from build123d import *

# Parameters (mm, degrees)
SKETCH1_W           = 110
SKETCH1_H           = 130
BOSS_EXTRUDE1_DEPTH = 4
SKETCH2_R           = 4.5
CUT_EXTRUDE1_DEPTH  = 4
SKETCH4_R           = 2.15
CUT_EXTRUDE2_DEPTH  = 86.240835285
SKETCH5_R           = 2.15
CUT_EXTRUDE3_DEPTH  = 86.240835285


with BuildPart() as part:
    # Sketch1 → Boss-Extrude1 (new body)
    with BuildSketch(Plane.XY):
        Rectangle(SKETCH1_W, SKETCH1_H)
    extrude(amount=BOSS_EXTRUDE1_DEPTH)

    # Sketch2 → Cut-Extrude1 (cut)
    with BuildSketch(Plane.XY.offset(4)):
        with Locations((0, 34.993291231)):
            Circle(SKETCH2_R)
    extrude(amount=-CUT_EXTRUDE1_DEPTH, mode=Mode.SUBTRACT)

    # Sketch4 → Cut-Extrude2 (cut, through all)
    with BuildSketch(Plane.XY.offset(4)):
        with Locations((-45.36112854, -47.475954891)):
            Circle(SKETCH4_R)
    extrude(amount=-CUT_EXTRUDE2_DEPTH, mode=Mode.SUBTRACT)

    # Sketch5 → Cut-Extrude3 (cut, through all)
    with BuildSketch(Plane.XY.offset(4)):
        with Locations((45.36112854, -47.475954891)):
            Circle(SKETCH5_R)
    extrude(amount=-CUT_EXTRUDE3_DEPTH, mode=Mode.SUBTRACT)


solid = part.part
Geometry: final body of the model. Coordinates: model frame, mm. Give positions to 0.01 mm unless a question says otherwise; leave off trailing zeros. Write each loop counter-clockwise with the first axis right and the second up, starting at its lowest first coordinate (ties: lowest second). Pieces come first, ordered by that corner, then holes. Notation, with made-up numbers: (-21.5, 9.25) -> (28.5, 9.25) arc R18 ccw to (28.5, 20.25) -> close; hole circle Ø5 at (88, 36). An arc over 180 degrees is marked (long way). Answer in a Markdown table with one row per item.
(1) Section query B-B on x = 46. Return loops of the section in (y, z).
Answers below:
| item | result |
|---|---|
| outline | (-65, 0) -> (-49.53, 0) -> (-49.53, 4) -> (-65, 4) -> close; (-45.42, 0) -> (65, 0) -> (65, 4) -> (-45.42, 4) -> close |
(2) Section query A-A on x = 0. Return loops of the section in (y, z), then the cut area to 3 significant figures.
Answers below:
| item | result |
|---|---|
| outline | (-65, 0) -> (30.49, 0) -> (30.49, 4) -> (-65, 4) -> close; (39.49, 0) -> (65, 0) -> (65, 4) -> (39.49, 4) -> close |
| area | 484 mm^2 |
(3) Ray query, line 1 along Y through (x, z) = (-45.5, 0.7); line 2 along X through (y, z) = (35, 0.85); line 3 along Y through (x, z) = (-3.5, 3). Return the intervals inside material, ascending. Write a range as [from, to].
Answers below:
| item | result |
|---|---|
| line 1 | [-65, -49.62], [-45.33, 65] |
| line 2 | [-55, -4.5], [4.5, 55] |
| line 3 | [-65, 32.16], [37.82, 65] |
(4) Draft query along X for faces 1 (the flat face through (-55, -1, 2)), 2 (the cylindrical face through (43.213, -47.381, 2.028)), 3 (the cylindrical face through (-0.98, 30.6, 2.03)), 4 (the flat face through (55, -1, 2)). Return one class per face: +X half, -X half, draft (parallel to the pull), parting line (faces both ways), or undercut.
Answers below:
| item | result |
|---|---|
| face 1 | -X half |
| face 2 | undercut |
| face 3 | undercut |
| face 4 | +X half |
